from build123d import *

# Parameters (mm, degrees)
F0_W     = 344.9914
F0_H     = 215.9
F0_R     = 31.75
F1_DEPTH = 9.525


# Not quite as in the source:
# - a length typed as a fraction of an inch, garbled in the dataset ("3 / 203.2 mm" for 3/8 in), is restored


with BuildPart() as f1:
    # F0 (on Top) → F1 (new body)
    with BuildSketch(Plane.XY):
        with Locations((0.0043, -50.8)):
            Rectangle(F0_W, F0_H)
        with BuildLine():
            ThreePointArc((-34.9247077073, -22.903081011), (-31.7715410013, -19.685073074), (-28.575, -22.86))
            Line((-28.575, -22.86), (-28.575, -31.75))
            ThreePointArc((-28.575, -31.75), (-31.7500524496, -34.9249999996), (-34.9249999983, -31.7498951008))
            Line((-34.9249999983, -31.7498951008), (-34.9247077073, -22.903081011))
        make_face(mode=Mode.SUBTRACT)
        Circle(F0_R, mode=Mode.SUBTRACT)
        with BuildLine():
            Line((-28.575, 40.64), (-28.575, 31.75))
            ThreePointArc((-28.575, 31.75), (-31.7500524496, 28.5750000004), (-34.9249999983, 31.7501048992))
            Line((-34.9249999983, 31.7501048992), (-34.9247077073, 40.596918989))
            ThreePointArc((-34.9247077073, 40.596918989), (-31.7715410013, 43.814926926), (-28.575, 40.64))
        make_face(mode=Mode.SUBTRACT)
        with BuildLine():
            ThreePointArc((28.5752922927, -22.903081011), (31.7284589987, -19.685073074), (34.925, -22.86))
            Line((34.925, -22.86), (34.925, -31.75))
            ThreePointArc((34.925, -31.75), (31.7499475504, -34.9249999996), (28.5750000017, -31.7498951008))
            Line((28.5750000017, -31.7498951008), (28.5752922927, -22.903081011))
        make_face(mode=Mode.SUBTRACT)
        with BuildLine():
            ThreePointArc((28.5752922927, 40.596918989), (31.7284589987, 43.814926926), (34.925, 40.64))
            Line((34.925, 40.64), (34.925, 31.75))
            ThreePointArc((34.925, 31.75), (31.7499475504, 28.5750000004), (28.5750000017, 31.7501048992))
            Line((28.5750000017, 31.7501048992), (28.5752922927, 40.596918989))
        make_face(mode=Mode.SUBTRACT)
    extrude(amount=F1_DEPTH)


solid = f1.part
Work out the finished part from the listing and answer in its coordinate system (mm). A direction names the side the tool comes from. Round coordinates to 2 decimals unless told otherwise and drop trailing zeros. Loops run counter-clockwise (first coordinate to the right, second up) from the corner with the lowest first, then second, coordinate; pieces in that order, holes last. Notation, with made-up numbers: (-14, -18.75) - (6, -18.75) arc R27 cw to (6, 17.25) - close; hole circle Ø11 at (20, 83). An arc over 180 degrees is marked (long way). Use one line per item in the form item = value. Start each with the question number.
(1) Find section C-C on z = 3.75. Determine the outline of the cut face in (x, y) (3 decimals).
(2) Which of the six approach directions +Z, -Z, +X, -X, +Y, -Y give full straight-line access (tool end or side, diameter ignored) to faces 5 (the face through (34.925, -27, 5)), 6 (the face through (-2, -49, 9.525))?
(3) Find section B-B on y = 0. Determine the outline of the cut face in (x, z) (3 decimals), and give its area (3 significant figures).
(4) Consider line 1 (Y direction, x = 0, z = 5.75); line 2 (X direction, y = -7, z = 5.5); line 3 (Y direction, x = 19, z = 8.75). Determine where each line is inside the solid, lowest interval first.
(5) Determine the mould class of faces 1 (the face through (-2, 57.15, 5)), 2 (the face through (-172.491, -52, 5)), 3 (the face through (-2, -158.75, 5)), 4 (the face through (-28.575, 36, 5)) for opening direction Y: +Y half, -Y half, draft (parallel to the pull), parting line (faces both ways), or undercut.
(6) Find section A-A on x = 0. Determine the outline of the cut face in (y, z) (3 decimals).
(7) Find section D-D on y = -27. Determine the outline of the cut face in (x, z) (3 decimals), and give its area (3 significant figures).
Answer list:
q1.outline = (-172.491, -158.75) - (172.5, -158.75) - (172.5, 57.15) - (-172.491, 57.15) - close; hole (-34.925, -31.75) arc R3.175 ccw to (-28.575, -31.75) - (-28.575, -22.86) arc R3.175 ccw (long way) to (-34.925, -22.903) - close; hole (-34.925, 31.75) arc R3.175 ccw to (-28.575, 31.75) - (-28.575, 40.64) arc R3.175 ccw (long way) to (-34.925, 40.597) - close; hole circle Ø63.5 at (0, 0); hole (28.575, -31.75) arc R3.175 ccw to (34.925, -31.75) - (34.925, -22.86) arc R3.175 ccw (long way) to (28.575, -22.903) - close; hole (28.575, 31.75) arc R3.175 ccw to (34.925, 31.75) - (34.925, 40.64) arc R3.175 ccw (long way) to (28.575, 40.597) - close
q2.face_5 = +Z, -Z
q2.face_6 = +Z, +X, -X, +Y, -Y
q3.outline = (-172.491, 0) - (-31.75, 0) - (-31.75, 9.525) - (-172.491, 9.525) - close; (31.75, 0) - (172.5, 0) - (172.5, 9.525) - (31.75, 9.525) - close
q3.area = 2,680 mm^2
q4.line_1 = -158.75 to -31.75, 31.75 to 57.15
q4.line_2 = -172.49 to -30.97, 30.97 to 172.5
q4.line_3 = -158.75 to -25.44, 25.44 to 57.15
q5.face_1 = +Y half
q5.face_2 = draft
q5.face_3 = -Y half
q5.face_4 = undercut
q6.outline = (-158.75, 0) - (-31.75, 0) - (-31.75, 9.525) - (-158.75, 9.525) - close; (31.75, 0) - (57.15, 0) - (57.15, 9.525) - (31.75, 9.525) - close
q7.outline = (-172.491, 0) - (-34.925, 0) - (-34.925, 9.525) - (-172.491, 9.525) - close; (-28.575, 0) - (-16.705, 0) - (-16.705, 9.525) - (-28.575, 9.525) - close; (16.705, 0) - (28.575, 0) - (28.575, 9.525) - (16.705, 9.525) - close; (34.925, 0) - (172.5, 0) - (172.5, 9.525) - (34.925, 9.525) - close
q7.area = 2,850 mm^2
